```python
from build123d import *

# Parameters (mm, degrees)
SKETCH2_R           = 8.636
SKETCH2_R_2         = 5.461
BOSS_EXTRUDE1_DEPTH = 820
FILLET1_R           = 1.016


with BuildPart() as part:
    # Sketch2 → Boss-Extrude1 (new body)
    with BuildSketch(Plane.XY):
        with Locations(Location((0, 0, 0), (0, 0, 180))):
            Circle(SKETCH2_R)
        with Locations(Location((0, 0, 0), (0, 0, 180))):
            Circle(SKETCH2_R_2, mode=Mode.SUBTRACT)
    extrude(amount=BOSS_EXTRUDE1_DEPTH)

    # Fillet1
    fillet1_edges = [part.edges().sort_by_distance(p)[0] for p in [
        (8.636, 0, 0),
        (8.636, 0, 820),
        (5.461, 0, 0),
        (5.461, 0, 820),
    ]]
    fillet(fillet1_edges, radius=FILLET1_R)


solid = part.part
```
Build history of the part. All positions in model axes, mm. Round coordinates to 2 decimals unless told otherwise and drop trailing zeros. Loops run counter-clockwise (first coordinate to the right, second up) from the corner with the lowest first, then second, coordinate; pieces in that order, holes last.
Item 1: Saw through at A-A (y = 0). List the corners of the cut face in (x, z).
Item 2: Saw through at C-C (z = 349). List the corners of the cut face in (x, y).
Item 3: Pin check, flat tips, straight feed: P1, Ø5, axis at x = 4.5, z = 168, coming from the -Y side; P2, Ø10, axis at x = 0, y = 0, coming from the +Z side; P3, Ø1.5, axis at x = 6.5, z = 413.5, coming from the +Y side; P4, Ø1, axis at y = -2, z = 91.5, coming from the +X side. Stop position of each tip, or through.
Item 4: Drill centre lines: line 1 along Y through (x, z) = (0, 573); line 2 along Y through (x, z) = (-1, 410); line 3 along X through (y, z) = (5, 101). Where is each one in solid material? Low to high.
Worked answers:
1. outline: (-8.64, 1.02) arc R1.02 ccw to (-7.62, 0) - (-6.48, 0) arc R1.02 ccw to (-5.46, 1.02) - (-5.46, 818.98) arc R1.02 ccw to (-6.48, 820) - (-7.62, 820) arc R1.02 ccw to (-8.64, 818.98) - close; (5.46, 1.02) arc R1.02 ccw to (6.48, 0) - (7.62, 0) arc R1.02 ccw to (8.64, 1.02) - (8.64, 818.98) arc R1.02 ccw to (7.62, 820) - (6.48, 820) arc R1.02 ccw to (5.46, 818.98) - close
2. outline: circle Ø17.27 at (0, 0); hole circle Ø10.92 at (0, 0)
3. P1: stops at y = -8.4
3. P2: passes through
3. P3: stops at y = 6.44
3. P4: stops at x = 8.5
4. line 1: y = -8.64 to -5.46, 5.46 to 8.64
4. line 2: y = -8.58 to -5.37, 5.37 to 8.58
4. line 3: x = -7.04 to -2.2, 2.2 to 7.04
